```python
from build123d import *

# Parameters (mm, degrees)
F0_R     = 18.5
F0_R_2   = 1.5
F0_R_3   = 6
F0_R_4   = 3
F1_DEPTH = 24
F2_DEPTH = 21.5
F3_DEPTH = 6
F5_DEPTH = 12
F7_DEPTH = 22.7


with BuildPart() as f1:
    # F0 (on Front) → F1 (new body)
    with BuildSketch(Plane.XZ):
        Circle(F0_R)
        with Locations((-7.75, -13.4233937587)):
            Circle(F0_R_2, mode=Mode.SUBTRACT)
        with Locations((7.75, -13.4233937587)):
            Circle(F0_R_2, mode=Mode.SUBTRACT)
        with Locations((-15.5, 0)):
            Circle(F0_R_2, mode=Mode.SUBTRACT)
        with Locations((-7.75, 13.4233937587)):
            Circle(F0_R_2, mode=Mode.SUBTRACT)
        with Locations((0, 7)):
            Circle(F0_R_3, mode=Mode.SUBTRACT)
        with Locations((15.5, 0)):
            Circle(F0_R_2, mode=Mode.SUBTRACT)
        with Locations((7.75, 13.4233937587)):
            Circle(F0_R_2, mode=Mode.SUBTRACT)
        with Locations((0, 7)):
            Circle(F0_R_3)
        with Locations((0, 7)):
            Circle(F0_R_4, mode=Mode.SUBTRACT)
        with Locations((0, 7)):
            Circle(F0_R_4)
    extrude(amount=F1_DEPTH)

    # F0 (on Front) → F2 (join)
    with BuildSketch(Plane.XZ):
        with Locations((0, 7)):
            Circle(F0_R_4)
    extrude(amount=-F2_DEPTH)

    # F0 (on Front) → F3 (join)
    with BuildSketch(Plane.XZ):
        with Locations((0, 7)):
            Circle(F0_R_3)
        with Locations((0, 7)):
            Circle(F0_R_4, mode=Mode.SUBTRACT)
    extrude(amount=-F3_DEPTH)

    # F4 (on face) → F5 (cut)
    with BuildSketch(Plane(origin=(0, 21.5, 0), x_dir=(-1, 0, 0), z_dir=(0, 1, 0))):
        with BuildLine():
            ThreePointArc((1.6583123952, 9.5), (0, 10), (-1.6583123952, 9.5))
            Line((-1.6583123952, 9.5), (1.6583123952, 9.5))
        make_face()
        with BuildLine():
            Line((-2, 10.5), (-2, 9.5))
            Line((-2, 9.5), (-1.6583123952, 9.5))
            ThreePointArc((-1.6583123952, 9.5), (0, 10), (1.6583123952, 9.5))
            Line((1.6583123952, 9.5), (2, 9.5))
            Line((2, 9.5), (2, 10.5))
            Line((2, 10.5), (-2, 10.5))
        make_face()
    extrude(amount=-F5_DEPTH, mode=Mode.SUBTRACT)

    # F6 (on face) → F7 (join)
    with BuildSketch(Plane.XZ.offset(24)):
        with BuildLine():
            ThreePointArc((16.4596774194, -1.1528309723), (14, 0), (16.4596774194, 1.1528309723))
            ThreePointArc((16.4596774194, 1.1528309723), (14.2894191624, 8.25), (9.228219618, 13.6780832971))
            ThreePointArc((9.228219618, 13.6780832971), (9.2445449854, 13.5512033299), (9.25, 13.4233937587))
            ThreePointArc((9.25, 13.4233937587), (6.8920411717, 12.1929846198), (7.2314578014, 14.8309142694))
            ThreePointArc((7.2314578014, 14.8309142694), (0, 16.5), (-7.2314578014, 14.8309142694))
            ThreePointArc((-7.2314578014, 14.8309142694), (-6.5195908611, 14.2813525869), (-6.25, 13.4233937587))
            ThreePointArc((-6.25, 13.4233937587), (-7.8778095713, 11.9288487732), (-9.228219618, 13.6780832971))
            ThreePointArc((-9.228219618, 13.6780832971), (-14.2894191624, 8.25), (-16.4596774194, 1.1528309723))
            ThreePointArc((-16.4596774194, 1.1528309723), (-14.8634138428, 1.3582187101), (-14, 0))
            ThreePointArc((-14, 0), (-14.8634138428, -1.3582187101), (-16.4596774194, -1.1528309723))
            ThreePointArc((-16.4596774194, -1.1528309723), (-14.2894191624, -8.25), (-9.228219618, -13.6780832971))
            ThreePointArc((-9.228219618, -13.6780832971), (-7.8778095713, -11.9288487732), (-6.25, -13.4233937587))
            ThreePointArc((-6.25, -13.4233937587), (-6.5195908611, -14.2813525869), (-7.2314578014, -14.8309142694))
            ThreePointArc((-7.2314578014, -14.8309142694), (0, -16.5), (7.2314578014, -14.8309142694))
            ThreePointArc((7.2314578014, -14.8309142694), (6.8920411717, -12.1929846198), (9.25, -13.4233937587))
            ThreePointArc((9.25, -13.4233937587), (9.2445449854, -13.5512033299), (9.228219618, -13.6780832971))
            ThreePointArc((9.228219618, -13.6780832971), (14.2894191624, -8.25), (16.4596774194, -1.1528309723))
        make_face()
        with BuildLine():
            ThreePointArc((9.25, 13.4233937587), (9.2445449854, 13.5512033299), (9.228219618, 13.6780832971))
            ThreePointArc((9.228219618, 13.6780832971), (8.25, 14.2894191624), (7.2314578014, 14.8309142694))
            ThreePointArc((7.2314578014, 14.8309142694), (6.8920411717, 12.1929846198), (9.25, 13.4233937587))
        make_face()
        with BuildLine():
            ThreePointArc((-6.25, 13.4233937587), (-6.5195908611, 14.2813525869), (-7.2314578014, 14.8309142694))
            ThreePointArc((-7.2314578014, 14.8309142694), (-8.25, 14.2894191624), (-9.228219618, 13.6780832971))
            ThreePointArc((-9.228219618, 13.6780832971), (-7.8778095713, 11.9288487732), (-6.25, 13.4233937587))
        make_face()
        with BuildLine():
            ThreePointArc((16.4596774194, -1.1528309723), (16.4899162736, -0.5767679692), (16.5, 0))
            ThreePointArc((16.5, 0), (16.4899162736, 0.5767679692), (16.4596774194, 1.1528309723))
            ThreePointArc((16.4596774194, 1.1528309723), (14, 0), (16.4596774194, -1.1528309723))
        make_face()
        with BuildLine():
            ThreePointArc((-14, 0), (-14.8634138428, 1.3582187101), (-16.4596774194, 1.1528309723))
            ThreePointArc((-16.4596774194, 1.1528309723), (-16.5, 0), (-16.4596774194, -1.1528309723))
            ThreePointArc((-16.4596774194, -1.1528309723), (-14.8634138428, -1.3582187101), (-14, 0))
        make_face()
        with BuildLine():
            ThreePointArc((-9.228219618, -13.6780832971), (-8.25, -14.2894191624), (-7.2314578014, -14.8309142694))
            ThreePointArc((-7.2314578014, -14.8309142694), (-6.5195908611, -14.2813525869), (-6.25, -13.4233937587))
            ThreePointArc((-6.25, -13.4233937587), (-7.8778095713, -11.9288487732), (-9.228219618, -13.6780832971))
        make_face()
        with BuildLine():
            ThreePointArc((7.2314578014, -14.8309142694), (8.25, -14.2894191624), (9.228219618, -13.6780832971))
            ThreePointArc((9.228219618, -13.6780832971), (9.2445449854, -13.5512033299), (9.25, -13.4233937587))
            ThreePointArc((9.25, -13.4233937587), (6.8920411717, -12.1929846198), (7.2314578014, -14.8309142694))
        make_face()
    extrude(amount=F7_DEPTH)


solid = f1.part
```
Geometry: final body of the model. Coordinates: model frame, mm. A direction names the side the tool comes from. Round coordinates to 2 decimals unless told otherwise and drop trailing zeros. Order: outer loops, then holes, each group sorted by start corner. A loop starts at its lowest first (then second) coordinate and runs counter-clockwise, first axis right, second up. Notation, with made-up numbers: (12, -20.5) -> (21, -20.5) arc R30 ccw to (21, 1.5) -> close; hole circle Ø6 at (-27, 37). An arc over 180 degrees is marked (long way). Use one line per item in the form item = value.
(1) Ray query, probe 1 along Z at (x, y) = (-7.75, -9.75); probe 2 along Z at (x, y) = (8.5, -9); probe 3 along X at (y, z) = (-36, -1). Return the intervals inside material, ascending. Write a range as [from, to].
Results list:
probe_1 = [-16.8, -14.92], [-11.92, 11.92], [14.92, 16.8]
probe_2 = [-16.43, -14.72], [-12.12, 12.12], [14.72, 16.43]
probe_3 = [-16.47, 16.47]
(2) Section C-C on z = -7.5. Return loops of the section in (x, y), and give its area (3 significant figures).
Results list:
outline = (-16.91, -24) -> (-14.7, -24) -> (-14.7, -46.7) -> (14.7, -46.7) -> (14.7, -24) -> (16.91, -24) -> (16.91, 0) -> (-16.91, 0) -> close
area = 1,480 mm^2
(3) Access query for faces 4 (the face through (0, 16, 9.5)), 5 (the face through (-6.9, -24, 15.2)), 6 (the face through (15, -24, 0)). Directions: +Z, -Z, +X, -X, +Y, -Y. A direction counts if a zero-diameter tool reaches every point of the face in a straight line with its end or side. Return the directions, or none.
Results list:
face_4 = +Z, +X, -X, +Y
face_5 = -Y
face_6 = +Y
(4) Section D-D on x = 8.5. Return loops of the section in (y, z), and give its area (3 significant figures).
Results list:
outline = (-46.7, -14.14) -> (-24, -14.14) -> (-24, -12.12) -> (0, -12.12) -> (0, 12.12) -> (-24, 12.12) -> (-24, 14.14) -> (-46.7, 14.14) -> close; (-24, -16.43) -> (0, -16.43) -> (0, -14.72) -> (-24, -14.72) -> close; (-24, 14.72) -> (0, 14.72) -> (0, 16.43) -> (-24, 16.43) -> close
area = 1,310 mm^2
(5) Draft query along X for faces 1 (the face through (14, -12, 0)), 2 (the face through (1, 6, 10)), 3 (the face through (-0.65, 13.64, 4.07)). Return one class per face: pulls with the +X half, pulls with the -X half, needs draft (parallel to the pull), parting line crosses it, or undercut.
Results list:
face_1 = undercut
face_2 = needs draft
face_3 = parting line crosses it
(6) Section B-B on y = -37. Return loops of the section in (x, z), and give its area (3 significant figures).
Results list:
outline = circle Ø33 at (0, 0)
area = 855 mm^2
(7) First-contact query: pin 1 Ø1.2 at (x, z) = (15.5, 0.5) entering from +Y; pin 2 Ø3 at (x, z) = (8, -13) entering from +Y; pin 3 Ø1.5 at (y, z) = (-10, 14.5) entering from -X. Flat tips, straight axial feed; report the tip coordinate or a pass-through.
Results list:
pin_1 = -24
pin_2 = 0
pin_3 = -12.38
(8) Section A-A on x = 0. Return loops of the section in (y, z).
Results list:
outline = (-46.7, -16.5) -> (-24, -16.5) -> (-24, -18.5) -> (0, -18.5) -> (0, 1) -> (6, 1) -> (6, 4) -> (21.5, 4) -> (21.5, 9.5) -> (9.5, 9.5) -> (9.5, 10) -> (6, 10) -> (6, 13) -> (0, 13) -> (0, 18.5) -> (-24, 18.5) -> (-24, 16.5) -> (-46.7, 16.5) -> close
